```python
from build123d import *

# Parameters (mm, degrees)
SKETCH_1_R               = 12.6
SKETCH_1_R_2             = 5.05
EXTRUDE_1_DEPTH          = 10
EXTRUDE_START            = -10
EXTRUDE_2_DEPTH          = 10
CUT_EXTRUDE_1_DEPTH      = 37.589103569
CUT_EXTRUDE_1_DEPTH_BACK = 37.589103569
SKETCH_3_R               = 1.45
CUT_EXTRUDE_2_DEPTH      = 37.589103725
CUT_EXTRUDE_2_DEPTH_BACK = 37.589103725
SKETCH_4_W               = 93.892826014
SKETCH_4_H               = 80.433232648
SKETCH_4_W_2             = 43.077359666
SKETCH_4_H_2             = 46.85


with BuildPart() as part:
    # 草图1 → 凸台-拉伸1 (new body)
    with BuildSketch(Plane.XY):
        with BuildLine():
            Line((-1.414911685, -15.535701623), (-1.414911685, -15.575321778))
            ThreePointArc((-1.414911685, -15.575321778), (0.005842023, -31.54999788), (1.403408047, -15.573276474))
            Line((1.403408047, -15.573276474), (1.403408047, -15.536745021))
            ThreePointArc((1.403408047, -15.536745021), (0.00577543, 15.599998931), (-1.414911685, -15.535701623))
        make_face()
        Circle(SKETCH_1_R, mode=Mode.SUBTRACT)
        with Locations((0, -23.5)):
            Circle(SKETCH_1_R_2, mode=Mode.SUBTRACT)
    extrude(amount=EXTRUDE_1_DEPTH)

    # 草图2 → 凸台-拉伸2 (add)
    with BuildSketch(Plane.XY.offset(10).offset(EXTRUDE_START)):
        Polygon((-14.77297225, -5.011914894), (-7.623232475, -26.086276596), (-5.929048094, -20.254331983), (0, -17.39919484), (5.929048094, -20.254331983), (7.623232475, -26.086276596), (14.77297225, -5.011914894), (5.311228847, -13.252346959), (0, -13.517472928), (-5.311228847, -13.252346959), align=None)
        with BuildLine():
            Line((-7.752949676, -16.366177664), (-7.630606655, -16.726792335))
            ThreePointArc((-7.630606655, -16.726792335), (-6.60716899, -17.691376281), (-5.234715693, -17.384425487))
            ThreePointArc((-5.234715693, -17.384425487), (-4.31764561, -16.705852785), (-3.31386093, -16.163732166))
            ThreePointArc((-3.31386093, -16.163732166), (-3.025346815, -15.633069871), (-3.458264207, -15.211850929))
            Line((-3.458264207, -15.211850929), (-4.103625329, -15.050589994))
            ThreePointArc((-4.103625329, -15.050589994), (-4.948227887, -14.794426004), (-5.776991612, -14.490906387))
            ThreePointArc((-5.776991612, -14.490906387), (-7.36504895, -14.796244404), (-7.752949676, -16.366177664))
        make_face(mode=Mode.SUBTRACT)
        with BuildLine():
            Line((4.103625329, -15.050589994), (3.458264207, -15.211850929))
            ThreePointArc((3.458264207, -15.211850929), (3.025346815, -15.633069871), (3.31386093, -16.163732166))
            ThreePointArc((3.31386093, -16.163732166), (4.31764561, -16.705852785), (5.234715693, -17.384425487))
            ThreePointArc((5.234715693, -17.384425487), (6.60716899, -17.691376281), (7.630606655, -16.726792335))
            Line((7.630606655, -16.726792335), (7.752949676, -16.366177664))
            ThreePointArc((7.752949676, -16.366177664), (7.36504895, -14.796244404), (5.776991612, -14.490906387))
            ThreePointArc((5.776991612, -14.490906387), (4.948227887, -14.794426004), (4.103625329, -15.050589994))
        make_face(mode=Mode.SUBTRACT)
    extrude(amount=EXTRUDE_2_DEPTH)

    # 草图3 → 切除-拉伸1 (cut, two sides: drawn at the far end of the back side and taken through both)
    with BuildSketch(Plane(origin=(0, 0, 0), x_dir=(1, 0, 0), z_dir=(0, 1, 0)).offset(-CUT_EXTRUDE_1_DEPTH_BACK)):
        with Locations(Location((0, -5, 0), (0, 0, 270))):
            Circle(SKETCH_3_R)
    extrude(amount=CUT_EXTRUDE_1_DEPTH + CUT_EXTRUDE_1_DEPTH_BACK, mode=Mode.SUBTRACT)

    # 草图4 → 切除-拉伸2 (cut, two sides: drawn at the far end of the back side and taken through both)
    with BuildSketch(Plane.XY.offset(10).offset(-CUT_EXTRUDE_2_DEPTH_BACK)):
        with Locations((-5.954078533, 0.891401237)):
            Rectangle(SKETCH_4_W, SKETCH_4_H)
        with Locations((3.186246386, -7.925)):
            Rectangle(SKETCH_4_W_2, SKETCH_4_H_2, mode=Mode.SUBTRACT)
    extrude(amount=CUT_EXTRUDE_2_DEPTH + CUT_EXTRUDE_2_DEPTH_BACK, mode=Mode.SUBTRACT)


solid = part.part
```
Source: CAD feature listing. Evaluate the final solid. Frame: model axes, mm. A direction names the side the tool comes from. Give positions to 0.01 mm unless a question says otherwise; leave off trailing zeros. Order: outer loops, then holes, each group sorted by start corner. A loop starts at its lowest first (then second) coordinate and runs counter-clockwise, first axis right, second up.
(1) Access query for faces 1 (the face through (0, -13, 0)), 2 (the face through (4.304, -16.697, 4.93)). Directions: +Z, -Z, +X, -X, +Y, -Y. A direction counts if a zero-diameter tool reaches every point of the face in a straight line with its end or side. Return the directions, or none.
(2) Section query C-C (z = 5). State how many separate pieces and enclosed holes the cut face has, plus the area to 3 significant figures.
(3) Material intervals for line 1 along Y through (x, z) = (0, 2.75); line 2 along Z through (x, y) = (0, -29.2); line 3 along Y through (x, z) = (4, 2.75), sorted ascending.
(4) Section query B-B (x = 0). Return the cut outline in (y, z).
(5) Pull-direction query (X, two-part tool) for faces 3 (the face through (3.02, -15.67, 4.93)), 4 (the face through (-1.6, 15.5, 4.9)), 5 (the face through (-9.999, -7.667, 4.93)), 6 (the face through (-5.432, -29.441, 4.93)); classes: +X half, -X half, draft (parallel to the pull), parting line (faces both ways), or undercut.
(6) Contact query for flat-ended pins moving along their axis: P1, Ø2, axis at x = 11.5, z = 2, coming from the +Y side; P2, Ø6, axis at x = -5, z = 6, coming from the +Y side; P3, Ø5, axis at x = -6.5, z = 7.5, coming from the +Y side. Output: stop coordinate, or through.
(7) Section query A-A (y = 0). Return the cut outline in (x, z), plus the area to 3 significant figures.
(8) Section query D-D (z = 7.5). Return the cut outline in (x, y).
Outcome:
1. face 1: -Z, +X, -X, +Y, -Y
1. face 2: +Z, -Z
2. separate pieces: 2
2. enclosed holes: 2
2. area: 433 mm2
3. line 1: y = -31.35 to -28.55, -18.45 to -12.6, 12.6 to 15.5
3. line 2: z = 0 to 3.55, 6.45 to 10
3. line 3: y = -30.49 to -26.58, -20.42 to -16.51, -15.08 to -11.95, 11.95 to 15.08
4. outline: (-31.35, 0) - (-28.55, 0) - (-28.55, 3.55) - (-31.35, 3.55) - close; (-31.35, 6.45) - (-28.55, 6.45) - (-28.55, 10) - (-31.35, 10) - close; (-18.45, 0) - (-12.6, 0) - (-12.6, 3.55) - (-18.45, 3.55) - close; (-18.45, 6.45) - (-12.6, 6.45) - (-12.6, 10) - (-18.45, 10) - close; (12.6, 0) - (15.5, 0) - (15.5, 3.55) - (12.6, 3.55) - close; (12.6, 6.45) - (15.5, 6.45) - (15.5, 10) - (12.6, 10) - close
5. face 3: undercut
5. face 4: draft
5. face 5: undercut
5. face 6: -X half
6. P1: stops at y = 11.54
6. P2: stops at y = 15.47
6. P3: stops at y = 15.08
7. outline: (-15.6, 0) - (-12.6, 0) - (-12.6, 10) - (-15.6, 10) - close; (12.6, 0) - (15.6, 0) - (15.6, 10) - (12.6, 10) - close
7. area: 60.0 mm2
8. outline: (-14.77, -5.01) - (-7.62, -26.09) arc R8.05 ccw to (-1.78, -31.35) - (1.78, -31.35) arc R8.05 ccw to (7.62, -26.09) - (14.77, -5.01) arc R15.6 ccw to (1.76, 15.5) - (-1.76, 15.5) arc R15.6 ccw to start; hole circle Ø25.2 at (0, 0); hole (-7.75, -16.37) - (-7.63, -16.73) arc R1.5 ccw to (-5.23, -17.38) arc R8.05 cw to (-3.31, -16.16) arc R0.5 ccw to (-3.36, -15.23) arc R15.6 cw to (-5.78, -14.49) arc R1.5 ccw to start; hole circle Ø10.1 at (0, -23.5); hole (3.31, -16.16) arc R8.05 cw to (5.23, -17.38) arc R1.5 ccw to (7.63, -16.73) - (7.75, -16.37) arc R1.5 ccw to (5.78, -14.49) arc R15.6 cw to (3.36, -15.23) arc R0.5 ccw to start
